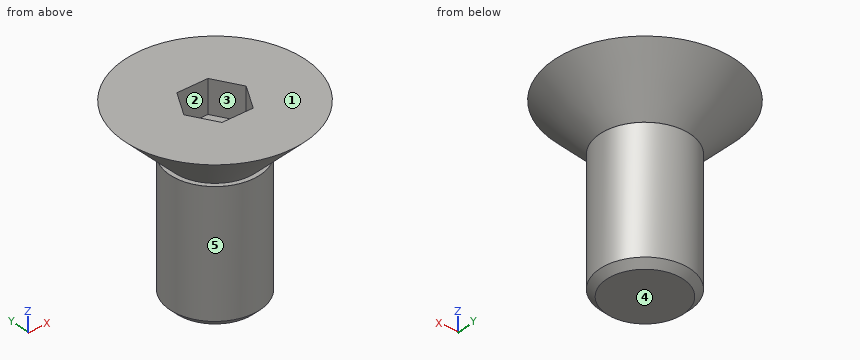
Solid Edge part; units mm, degrees
sketch "Sketch1" plane through (0, 0, 0) normal (0, 0, 1) x (1, 0, 0)
  circle A0 centre (0, 0) radius 10
extrude "Protrusion1" add sketch "Sketch1" along normal blind 5.5
sketch "Sketch2" plane through (0, 0, 0) normal (0, 0, -1) x (1, 0, 0)
  circle A0 centre (0, 0) radius 5
extrude "Protrusion2" add sketch "Sketch2" along normal blind 14.5
sketch "Sketch3" plane through (0, 0, -14.5) normal (0, 0, -1) x (1, 0, 0)
  circle A0 centre (0, 0) radius 4.9997
extrude "Cutout1" cut sketch "Sketch3" against normal blind 14.4855 flip side to cut
chamfer "Chamfer_1" distance 0.75 angle 45 1 edges at (-4.9997, 0, -14.5)
sketch "Sketch4" plane through (0, 0, 5.5) normal (0, 0, 1) x (1, 0, 0)
  line L0 (-1.7321, 3) -> (1.7321, 3)
  line L1 (3.4641, 0) -> (1.7321, 3)
  line L2 (1.7321, -3) -> (3.4641, 0)
  line L3 (-1.7321, -3) -> (1.7321, -3)
  line L4 (-3.4641, 0) -> (-1.7321, -3)
  line L5 (-1.7321, 3) -> (-3.4641, 0)
extrude "Cutout2" cut sketch "Sketch4" against normal blind 3.6667
sketch "Sketch5" plane through (0, 0, 0) normal (0, -1, 0) x (1, 0, 0)
  line L0 (10, 5.5) -> (4.5, 0)
  line L1 (4.5, 0) -> (10, 0)
  line L2 (10, 0) -> (10, 5.5)
revolve "RevolvedCutout1" cut sketch "Sketch5" angle 360 about axis through (0, 0, 14.0017) along (0, 0, -1)
properties part number "185736" material "Stainless Steel, 304"
Can you work these out from the model? Positions are in its coordinate system, mm. Face numbers are marked on the shaded views. A direction names the side the tool comes from. Coordinates: 2 decimals unless noted, no trailing zeros. Write each loop counter-clockwise with the first axis right and the second up, starting at its lowest first coordinate (ties: lowest second). Pieces come first, ordered by that corner, then holes. Notation, with made-up numbers: (69.5, -6) -> (118.5, -6) arc R20 ccw to (118.5, 19) -> close; hole circle Ø5 at (38, 15). An arc over 180 degrees is marked (long way). Write each question's results on one line, items separated by ' | '. Start each with the question number.
Q1. We'd pull the mould along X, two halves only. Please class the marked faces 3, 4 and 5: +X half, -X half, draft (parallel to the pull), parting line (faces both ways), or undercut.
Q2. Imagine slicing it at C-C (z = -10.75). Write out the boundary of the cut face in (x, y), then the cut area to 3 significant figures.
Q3. If I drill on probe 1 along X at (y, z) = (0.5, 3.5); probe 2 along Z at (x, y) = (-0.5, 2); probe 3 along Y at (x, z) = (0, -9), over which ranges is the centre line in solid material (lowest first)?
Q4. Imagine slicing it at A-A (z = 3). Write out the boundary of the cut face in (x, y).
Q5. I'm going to push flat-ended pins straight in: pin 1 (3 mm diameter, centred on x = 7, z = -8, fed in from +Y); pin 2 (8 mm diameter, centred on y = -4.5, z = -1, fed in from -X); pin 3 (2 mm diameter, centred on y = 4, z = -4, fed in from -X); pin 4 (8 mm diameter, centred on x = -1.5, y = -2, fed in from +Z). Where does each tip first touch, or does it pass through?
Q6. On a 3-axis mill with a long thin cutter (end or side, diameter ignored), from which of +Z, -Z, +X, -X, +Y, -Y can I reach the whole of each face in a straight line? I mean the marked faces 1 and 2. Say none if no direction works.
Taken from the geometry:
1) face 3: undercut | face 4: draft | face 5: parting line
2) outline: circle Ø10 at (0, 0) | area: 78.5 mm^2
3) probe 1: x = -7.98 to -3.18, 3.18 to 7.98 | probe 2: z = -14.5 to 1.83 | probe 3: y = -5 to 5
4) outline: circle Ø15 at (0, 0); hole (-3.46, 0) -> (-1.73, -3) -> (1.73, -3) -> (3.46, 0) -> (1.73, 3) -> (-1.73, 3) -> close
5) pin 1: passes through | pin 2: stops at x = -6.55 | pin 3: stops at x = -4 | pin 4: stops at z = 5.5
6) face 1: +Z, +X, -X, +Y, -Y | face 2: +Z
